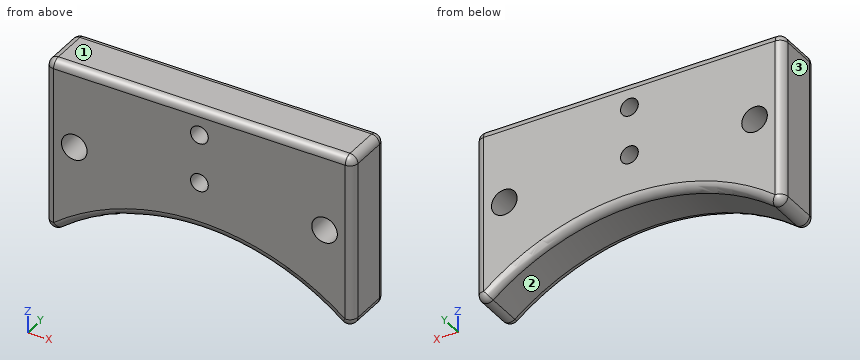
```python
from build123d import *

# Parameters (mm, degrees)
F0_R     = 3.25
F0_R_2   = 2.25
F1_DEPTH = 13
F2_R     = 2
F3_R     = 2


with BuildPart() as f1:
    # F0 (on Front) → F1 (new body)
    with BuildSketch(Plane.XZ):
        with BuildLine():
            Line((-39, 0), (-39, -46))
            ThreePointArc((-39, -46), (0, -31), (39, -46))
            Line((39, -46), (39, 0))
            Line((39, 0), (-39, 0))
        make_face()
        with Locations((-31.75, -20.5)):
            Circle(F0_R, mode=Mode.SUBTRACT)
        with Locations((0, -18.95)):
            Circle(F0_R_2, mode=Mode.SUBTRACT)
        with Locations((31.75, -20.5)):
            Circle(F0_R, mode=Mode.SUBTRACT)
        with Locations((0, -6.65)):
            Circle(F0_R_2, mode=Mode.SUBTRACT)
    extrude(amount=-F1_DEPTH)

    # F2
    f2_edges = [f1.edges().sort_by_distance(p)[0] for p in [
        (-39, 6.5, -46),
        (39, 6.5, -46),
    ]]
    fillet(f2_edges, radius=F2_R)

    # F3
    f3_edges = [f1.edges().sort_by_distance(p)[0] for p in [
        (-39, 6.5, 0),
        (39, 6.5, 0),
        (0, 0, 0),
        (0, 13, 0),
        (-39, 0, -20.856369),
        (-39, 6.5, -41.712739),
        (-39, 13, -20.856369),
    ]]
    fillet(f3_edges, radius=F3_R)


solid = f1.part
```
Build history of the part. All positions in model axes, mm. Face numbers are marked on the shaded views. Round coordinates to 2 decimals unless told otherwise and drop trailing zeros. Order: outer loops, then holes, each group sorted by start corner. A loop starts at its lowest first (then second) coordinate and runs counter-clockwise, first axis right, second up. Notation, with made-up numbers: (-22, -34.75) - (8, -34.75) arc R31 ccw to (8, -0.75) - close; hole circle Ø10 at (-25.75, 11.5). An arc over 180 degrees is marked (long way). Use a Markdown table: item, result.
1) Saw through at A-A on z = -6.65. Write the cut outline in (x, y), and give its area (3 significant figures).
Recorded:
| item | result |
|---|---|
| outline | (-39, 2) arc R2 ccw to (-37, 0) - (-2.25, 0) - (-2.25, 13) - (-37, 13) arc R2 ccw to (-39, 11) - close; (2.25, 0) - (37, 0) arc R2 ccw to (39, 2) - (39, 11) arc R2 ccw to (37, 13) - (2.25, 13) - close |
| area | 952 mm² |
2) Flat gauge pin, fed straight in: pin 1 Ø2 at (x, y) = (-23.5, 11) entering from -Z. Where does the tip first touch, or does it go through?
Recorded:
| item | result |
|---|---|
| pin 1 | stops at z = -36.41 |
3) Pull direction X, two halves, no side cores. Call the marked faces 1, 2 and 3: pulls with the +X half, pulls with the -X half, needs draft (parallel to the pull), parting line crosses it, or undercut.
Recorded:
| item | result |
|---|---|
| face 1 | needs draft |
| face 2 | undercut |
| face 3 | pulls with the -X half |
4) Saw through at D-D on z = -18.95. Write the cut outline in (x, y), and give its area (3 significant figures).
Recorded:
| item | result |
|---|---|
| outline | (-39, 2) arc R2 ccw to (-37, 0) - (-34.61, 0) - (-34.61, 13) - (-37, 13) arc R2 ccw to (-39, 11) - close; (-28.89, 0) - (-2.25, 0) - (-2.25, 13) - (-28.89, 13) - close; (2.25, 0) - (28.89, 0) - (28.89, 13) - (2.25, 13) - close; (34.61, 0) - (37, 0) arc R2 ccw to (39, 2) - (39, 11) arc R2 ccw to (37, 13) - (34.61, 13) - close |
| area | 804 mm² |
5) Saw through at C-C on y = 3.25. Write the cut outline in (x, z), and give its area (3 significant figures).
Recorded:
| item | result |
|---|---|
| outline | (-39, -41.71) arc R2 ccw to (-35.77, -43.29) arc R58.2 cw to (35.77, -43.29) arc R2 ccw to (39, -41.71) - (39, -2) arc R2 ccw to (37, 0) - (-37, 0) arc R2 ccw to (-39, -2) - close; hole circle Ø6.5 at (-31.75, -20.5); hole circle Ø4.5 at (0, -18.95); hole circle Ø4.5 at (0, -6.65); hole circle Ø6.5 at (31.75, -20.5) |
| area | 2,680 mm² |
6) Wall check: L1, parallel to Z at x = 0, y = 3.25; L2, parallel to X at y = 2, z = -17.5; L3, parallel to X at y = 7.5, z = -6.5 (3 decimals). Give the ranges that are in metal, low to high.
Recorded:
| item | result |
|---|---|
| L1 | z = -31 to -21.2, -16.7 to -8.9, -4.4 to 0 |
| L2 | x = -39 to -33, -30.5 to -1.72, 1.72 to 30.5, 33 to 39 |
| L3 | x = -39 to -2.245, 2.245 to 39 |
7) Saw through at B-B on x = 0. Write the cut outline in (y, z), and give its area (3 significant figures).
Recorded:
| item | result |
|---|---|
| outline | (0, -29) arc R2 ccw to (2, -31) - (11, -31) arc R2 ccw to (13, -29) - (13, -21.2) - (0, -21.2) - close; (0, -16.7) - (13, -16.7) - (13, -8.9) - (0, -8.9) - close; (0, -4.4) - (13, -4.4) - (13, -2) arc R2 ccw to (11, 0) - (2, 0) arc R2 ccw to (0, -2) - close |
| area | 283 mm² |
